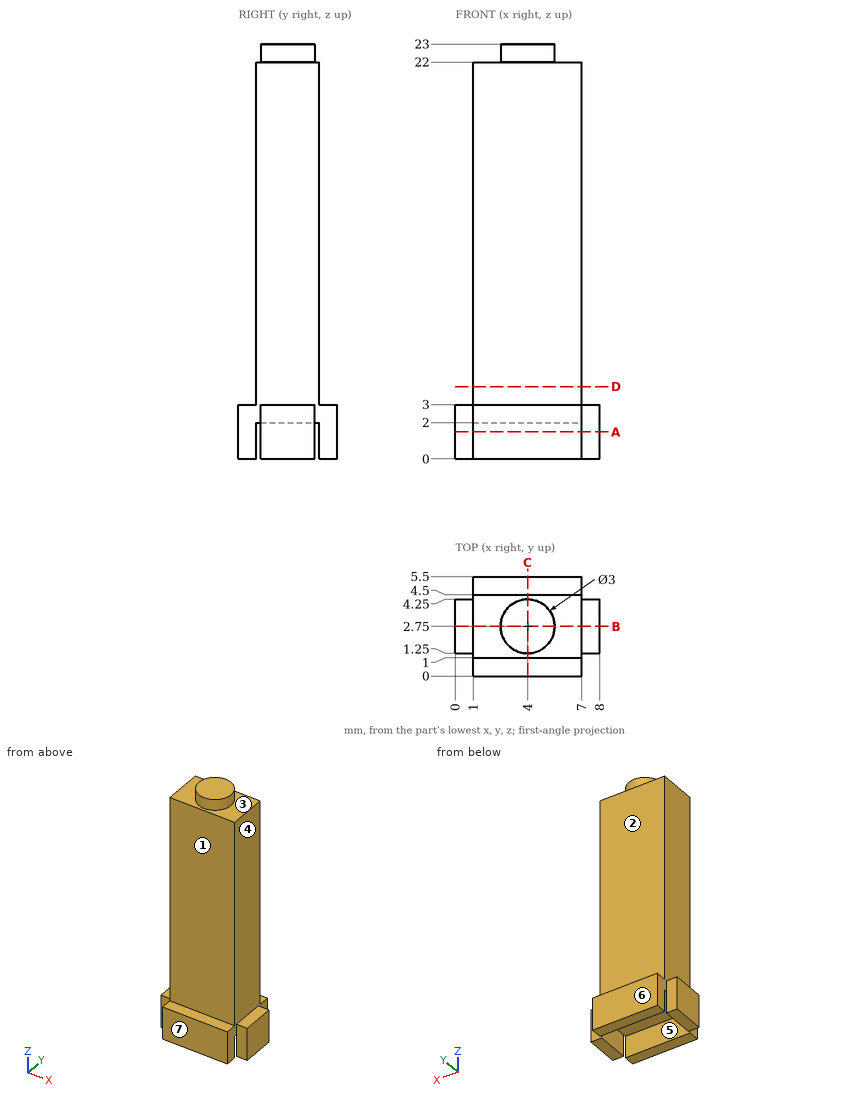
Input: dimensioned drawing with shaded views. Units: mm. Origin: part minimum x, y, z. A direction names the side the tool comes from. Round coordinates to 2 decimals unless told otherwise and drop trailing zeros. Order: outer loops, then holes, each group sorted by start corner. A loop starts at its lowest first (then second) coordinate and runs counter-clockwise, first axis right, second up. Notation, with made-up numbers: (17.25, 65.25) - (60.25, 65.25) arc R7 cw to (60.25, 74.25) - close; hole circle Ø6 at (41, 0). An arc over 180 degrees is marked (long way). Write item = value, one per line. Start each with the question number.
Q1. Access query for the marked faces 1, 2 and 3. Directions: +Z, -Z, +X, -X, +Y, -Y. A direction counts if a zero-diameter tool reaches every point of the face in a straight line with its end or side. Return the directions, or none.
Q2. Ray query, line 1 (Y direction, x = 3.25, z = 19.75); line 2 (X direction, y = 1.9, z = 17.5); line 3 (Z direction, x = 4, y = 1.9). Return the intervals inside material, ascending. Write a range as from..to.
Q3. Cut plane B-B on y = 2.75. Return the cut outline in (x, z).
Q4. Cut plane A-A on z = 1.5. Return the cut outline in (x, y).
Q5. Cut plane D-D on z = 4. Return the cut outline in (x, y).
Q6. Cut plane C-C on x = 4. Return the cut outline in (y, z).
Q7. Pin query (flat end, axial travel): pin 1 (1.8 mm diameter, centred on x = 3, z = 11, fed in from -Y); pin 2 (1.1 mm diameter, centred on x = 0.5, z = 2, fed in from -Y); pin 3 (0.8 mm diameter, centred on x = 7.5, z = 1, fed in from +Y); pin 4 (0.5 mm diameter, centred on x = 2.5, y = 0.5, fed in from +Z). Return the tip coordinate at first contact, or that it passes through.
Q8. Pull-direction query (Y, two-part tool) for the marked faces 4, 5, 6 and 7; classes: +Y half, -Y half, draft (parallel to the pull), parting line (faces both ways), or undercut.
Outcome:
q1.face_1 = +Z, +X, -X, -Y
q1.face_2 = +Z, +X, -X, +Y
q1.face_3 = +Z
q2.line_1 = 1..4.5
q2.line_2 = 1..7
q2.line_3 = 2..23
q3.outline = (0, 0) - (1, 0) - (1, 2) - (7, 2) - (7, 0) - (8, 0) - (8, 3) - (7, 3) - (7, 22) - (5.5, 22) - (5.5, 23) - (2.5, 23) - (2.5, 22) - (1, 22) - (1, 3) - (0, 3) - close
q4.outline = (0, 1.25) - (1, 1.25) - (1, 4.25) - (0, 4.25) - close; (1, 0) - (7, 0) - (7, 1) - (1, 1) - close; (1, 4.5) - (7, 4.5) - (7, 5.5) - (1, 5.5) - close; (7, 1.25) - (8, 1.25) - (8, 4.25) - (7, 4.25) - close
q5.outline = (1, 1) - (7, 1) - (7, 4.5) - (1, 4.5) - close
q6.outline = (0, 0) - (1, 0) - (1, 2) - (4.5, 2) - (4.5, 0) - (5.5, 0) - (5.5, 3) - (4.5, 3) - (4.5, 22) - (4.25, 22) - (4.25, 23) - (1.25, 23) - (1.25, 22) - (1, 22) - (1, 3) - (0, 3) - close
q7.pin_1 = 1
q7.pin_2 = 0
q7.pin_3 = 4.25
q7.pin_4 = 3
q8.face_4 = draft
q8.face_5 = undercut
q8.face_6 = +Y half
q8.face_7 = -Y half
